Here's how the part is built. I have some questions about the finished solid (model axes, mm). A direction names the side the tool comes from. Round coordinates to 2 decimals unless told otherwise and drop trailing zeros. Write each loop counter-clockwise with the first axis right and the second up, starting at its lowest first coordinate (ties: lowest second). Pieces come first, ordered by that corner, then holes. Notation, with made-up numbers: (7.25, -39.75) - (14.25, -39.75) arc R12 ccw to (14.25, -35.75) - close; hole circle Ø3 at (66.25, 19.25). An arc over 180 degrees is marked (long way). Use one line per item in the form item = value. Start each with the question number.
1. Which directions (+Z, -Z, +X, -X, +Y, -Y) give clear straight access to the entire face, cutting with the end or side of a thin tool? Please do faces 1 (the flat face through (9.5, 19.1, 1.5)), 2 (the cylindrical face through (42.645, 13.062, 1.479)), 3 (the cylindrical face through (32.355, 61.938, 1.479)), 4 (the cylindrical face through (49.77, 69.32, 1.48)).
2. I want a section at B-B, the plane x = 37.5. List the corners of the cut face in (y, z) for me.
3. If I drill on line 1 along Y through (x, z) = (49, 1.05); line 2 along Y through (x, z) = (37.5, 1.15); line 3 along Y through (x, z) = (50, 0.85), over which ranges is the centre line in solid material (lowest first)?
4. We'd pull the mould along Y, two halves only. Please class faces 5 (the cylindrical face through (7.5, 60, 1.5)), 6 (the flat face through (55.9, 9.5, 1.5)), 7 (the cylindrical face through (61.938, 42.645, 1.479)), 8 (the flat face through (65.5, 55.9, 1.5)): +Y half, -Y half, draft (parallel to the pull), parting line (faces both ways), or undercut.
5. I want a section at A-A, the plane y = 6.5. List the corners of the cut face in (x, z) for me.
6. I want a section at C-C, the plane y = 33. List the corners of the cut face in (x, z) for me.
```python
from build123d import *

# Parameters (mm, degrees)
F0_R     = 3
F1_DEPTH = 3


with BuildPart() as f1:
    # F0 (on Top) → F1 (new body)
    with BuildSketch(Plane.XY):
        with BuildLine():
            ThreePointArc((57.3301127781, 5.6720778685), (67.5811295865, 15.1085810454), (73.679486557, 27.6361897588))
            ThreePointArc((73.679486557, 27.6361897588), (69.2456728253, 25.2293463411), (64.8118590936, 27.6361897588))
            ThreePointArc((64.8118590936, 27.6361897588), (63.5273534072, 32.1621670241), (59.5437049903, 34.6651593043))
            ThreePointArc((59.5437049903, 34.6651593043), (56.5473999136, 30.5977037223), (51.7587434047, 28.9881050568))
            ThreePointArc((51.7587434047, 28.9881050568), (43.2853466758, 36.2848022119), (49.588750459, 45.5209996029))
            ThreePointArc((49.588750459, 45.5209996029), (55.4595817481, 44.828212266), (59.4162546646, 40.4360199032))
            ThreePointArc((59.4162546646, 40.4360199032), (61.9654848992, 42.6842952192), (63.1107981169, 45.8845411972))
            Line((63.1107981169, 45.8845411972), (62.1492189347, 46.1509661226))
            Line((62.1492189347, 46.1509661226), (61.9658155367, 50.3289483488))
            Line((61.9658155367, 50.3289483488), (61.7824121386, 54.5069305749))
            Line((61.7824121386, 54.5069305749), (69.3279221315, 57.3301127781))
            ThreePointArc((69.3279221315, 57.3301127781), (59.8914189546, 67.5811295865), (47.3638102412, 73.679486557))
            ThreePointArc((47.3638102412, 73.679486557), (49.7706536589, 69.2456728253), (47.3638102412, 64.8118590936))
            ThreePointArc((47.3638102412, 64.8118590936), (42.8378329759, 63.5273534072), (40.3348406957, 59.5437049903))
            ThreePointArc((40.3348406957, 59.5437049903), (44.4022962777, 56.5473999136), (46.0118949432, 51.7587434047))
            ThreePointArc((46.0118949432, 51.7587434047), (46.012965743, 51.6813590294), (46.0133226864, 51.603968069))
            ThreePointArc((46.0133226864, 51.603968069), (38.6384185061, 43.2756291652), (29.4790003971, 49.588750459))
            ThreePointArc((29.4790003971, 49.588750459), (30.171787734, 55.4595817481), (34.5639800968, 59.4162546646))
            ThreePointArc((34.5639800968, 59.4162546646), (32.3157047808, 61.9654848992), (29.1154588028, 63.1107981169))
            Line((29.1154588028, 63.1107981169), (28.8490338774, 62.1492189347))
            Line((28.8490338774, 62.1492189347), (24.6710516512, 61.9658155367))
            Line((24.6710516512, 61.9658155367), (20.4930694251, 61.7824121386))
            Line((20.4930694251, 61.7824121386), (17.6698872219, 69.3279221315))
            ThreePointArc((17.6698872219, 69.3279221315), (7.4188704135, 59.8914189546), (1.320513443, 47.3638102412))
            ThreePointArc((1.320513443, 47.3638102412), (5.7543271747, 49.7706536589), (10.1881409064, 47.3638102412))
            ThreePointArc((10.1881409064, 47.3638102412), (11.4726465928, 42.8378329759), (15.4562950097, 40.3348406957))
            ThreePointArc((15.4562950097, 40.3348406957), (18.4526000864, 44.4022962777), (23.2412565953, 46.0118949432))
            ThreePointArc((23.2412565953, 46.0118949432), (29.2736601064, 43.6104288236), (31.786001315, 37.6233533025))
            ThreePointArc((31.786001315, 37.6233533025), (30.0028163347, 32.4520878764), (25.411249541, 29.4790003971))
            ThreePointArc((25.411249541, 29.4790003971), (19.5404182519, 30.171787734), (15.5837453354, 34.5639800968))
            ThreePointArc((15.5837453354, 34.5639800968), (13.0345151008, 32.3157047808), (11.8892018831, 29.1154588028))
            Line((11.8892018831, 29.1154588028), (12.8507810653, 28.8490338774))
            Line((12.8507810653, 28.8490338774), (13.0341844633, 24.6710516512))
            Line((13.0341844633, 24.6710516512), (13.2175878614, 20.4930694251))
            Line((13.2175878614, 20.4930694251), (5.6720778685, 17.6698872219))
            ThreePointArc((5.6720778685, 17.6698872219), (15.1085810454, 7.4188704135), (27.6361897588, 1.320513443))
            ThreePointArc((27.6361897588, 1.320513443), (25.2293463411, 5.7543271747), (27.6361897588, 10.1881409064))
            ThreePointArc((27.6361897588, 10.1881409064), (32.1621670241, 11.4726465928), (34.6651593043, 15.4562950097))
            ThreePointArc((34.6651593043, 15.4562950097), (30.5977037223, 18.4526000864), (28.9881050568, 23.2412565953))
            ThreePointArc((28.9881050568, 23.2412565953), (36.2848022119, 31.7146533242), (45.5209996029, 25.411249541))
            ThreePointArc((45.5209996029, 25.411249541), (45.7049856013, 24.4110971346), (45.7666160814, 23.396031931))
            ThreePointArc((45.7666160814, 23.396031931), (44.3070014429, 18.6672086771), (40.4360199032, 15.5837453354))
            ThreePointArc((40.4360199032, 15.5837453354), (42.6842952192, 13.0345151008), (45.8845411972, 11.8892018831))
            Line((45.8845411972, 11.8892018831), (46.1509661226, 12.8507810653))
            Line((46.1509661226, 12.8507810653), (50.3289483488, 13.0341844633))
            Line((50.3289483488, 13.0341844633), (54.5069305749, 13.2175878614))
            Line((54.5069305749, 13.2175878614), (57.3301127781, 5.6720778685))
        make_face()
        with Locations((37.5, 37.5)):
            Circle(F0_R, mode=Mode.SUBTRACT)
    extrude(amount=F1_DEPTH)


solid = f1.part
```
Model answer:
q1.face_1 = +Z, -Z, -X
q1.face_2 = +Z, -Z, -Y
q1.face_3 = +Z, -Z, +Y
q1.face_4 = +Z, -Z
q2.outline = (31.79, 0) - (34.5, 0) - (34.5, 3) - (31.79, 3) - close; (40.5, 0) - (43.21, 0) - (43.21, 3) - (40.5, 3) - close
q3.line_1 = 12.98 to 29.4, 45.35 to 66.5, 71.99 to 73.19
q3.line_2 = 31.79 to 34.5, 40.5 to 43.21
q3.line_3 = 13.02 to 29.14, 45.61 to 72.86
q4.face_5 = +Y half
q4.face_6 = -Y half
q4.face_7 = undercut
q4.face_8 = undercut
q5.outline = (16.4, 0) - (25.28, 0) - (25.28, 3) - (16.4, 3) - close; (57.02, 0) - (58.6, 0) - (58.6, 3) - (57.02, 3) - close
q6.outline = (13.57, 0) - (16.39, 0) - (16.39, 3) - (13.57, 3) - close; (30.4, 0) - (44.45, 0) - (44.45, 3) - (30.4, 3) - close; (58.76, 0) - (62.78, 0) - (62.78, 3) - (58.76, 3) - close
